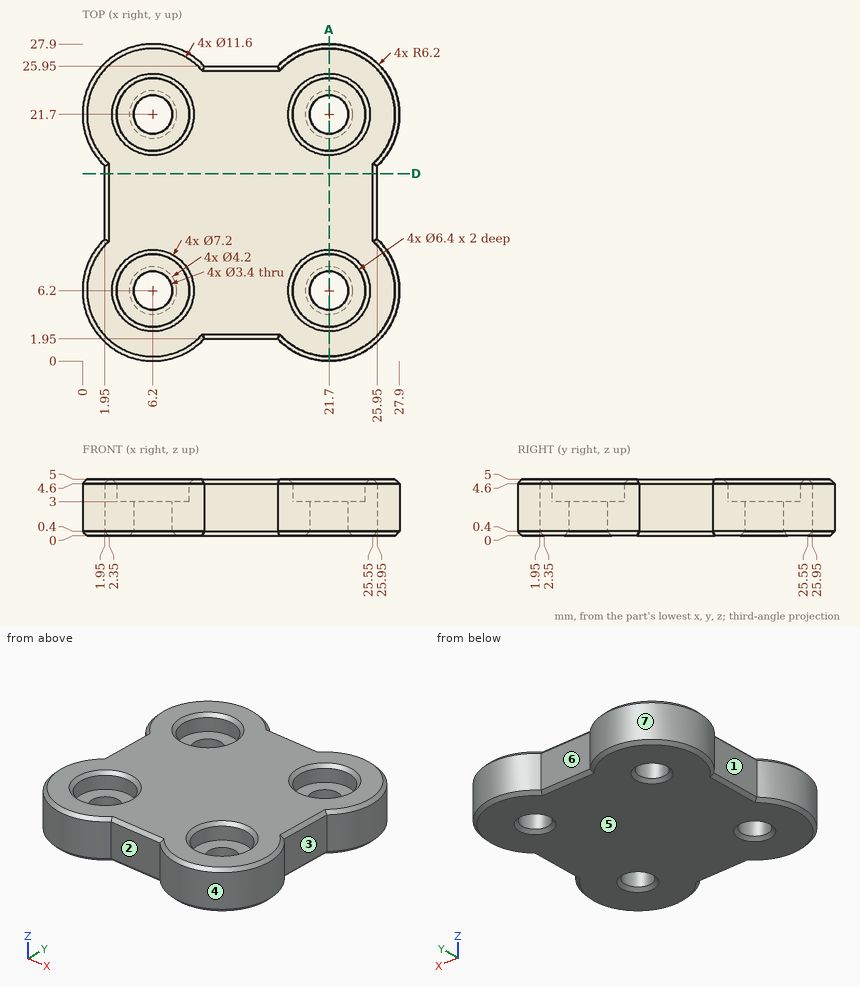
Job drawing, mm, ordinate dimensions from the low corner. One solid piece. A direction names the side the tool comes from. Coordinates: 2 decimals unless noted, no trailing zeros. Write each loop counter-clockwise with the first axis right and the second up, starting at its lowest first coordinate (ties: lowest second). Pieces come first, ordered by that corner, then holes. Notation, with made-up numbers: M -2,-20.5 L 6,-20.5 A21 cw 6,8.5 Z; hole C 38.5,47 d3. An arc over 180 degrees is marked long. Answer as a JSON object with one key per item and string values. Group by question number.
1) Saw through at A-A (x = 21.7). Give the number of separate pieces and of enclosed holes in the cut face, plus the area to 3 significant figures.
2) Tool access for the marked faces 1, 2 and 3: list every direction of +Z, -Z, +X, -X, +Y, -Y with a clear straight run to the whole face (end or side of a thin tool).
3) Saw through at D-D (y = 16.5). Write the cut outline in (x, z), plus the area to 3 significant figures.
4) Wall check: line 1 (Y direction, x = 6.2, z = 1.4); line 2 (Y direction, x = 21.7, z = 3.7). Give the ranges that are in metal, low to high. Write a range as from..to.
5) Mould opens along Y. For the marked faces 4, 5, 6 and 7 say: +Y half, -Y half, draft (parallel to the pull), parting line (faces both ways), or undercut.
6) Pin check, flat tips, straight feed: pin 1 Ø4 at (x, y) = (6.2, 6.2) entering from -Z; pin 2 Ø1.3 at (y, z) = (14, 1.5) entering from +X; pin 3 Ø2 at (x, z) = (4, 2) entering from -Y; pin 4 Ø2.5 at (x, y) = (21.7, 6.2) entering from -Z. Stop position of each tip, or through.
Values follow:
{
 "1": {"separate pieces": "3", "enclosed holes": "0", "area": "92.5 mm2"},
 "2": {"face 1": "+Z, -Z, -X", "face 2": "+Z, -Z, -Y", "face 3": "+Z, -Z, +X"},
 "3": {"outline": "M 1.95,0.4 L 2.35,0 L 25.55,0 L 25.95,0.4 L 25.95,4.6 L 25.55,5 L 2.35,5 L 1.95,4.6 Z", "area": "120 mm2"},
 "4": {"line 1": "y = 0..4.5, 7.9..20, 23.4..27.9", "line 2": "y = 0..3, 9.4..18.5, 24.9..27.9"},
 "5": {"face 4": "undercut", "face 5": "draft", "face 6": "+Y half", "face 7": "undercut"},
 "6": {"pin 1": "stops at z = 0.1", "pin 2": "stops at x = 25.95", "pin 3": "stops at y = 0.12", "pin 4": "passes through"}
}
